from build123d import *

# Parameters (mm, degrees)
F0_W     = 30.5993435904
F0_H     = 25.6396476179
F1_DEPTH = 40
F2_R     = 6.5677441637
F3_DEPTH = 25.6406476179
F4_R     = 5
F5_SIZE  = 5
F6_T     = -2.5


with BuildPart() as f1:
    # F0 (on Top) → F1 (new body)
    with BuildSketch(Plane.XY):
        with Locations((-1.0232594796, 2.7313483879)):
            Rectangle(F0_W, F0_H)
    extrude(amount=F1_DEPTH)

    # F2 (on face) → F3 (cut, through all)
    with BuildSketch(Plane.XZ.offset(10.0884754211)):
        with Locations((-5.0276978873, 21.8645650893)):
            Circle(F2_R)
    extrude(amount=-F3_DEPTH, mode=Mode.SUBTRACT)

    # F4
    f4_edges = [f1.edges().sort_by_distance(p)[0] for p in [
        (-1.023259, -10.088475, 40),
    ]]
    fillet(f4_edges, radius=F4_R)

    # F5
    f5_edges = [f1.edges().sort_by_distance(p)[0] for p in [
        (-1.023259, 15.551172, 40),
    ]]
    chamfer(f5_edges, length=F5_SIZE)

    # F6
    f6_openings = [f1.faces().sort_by_distance(p)[0] for p in [
        (-1.023259, 2.731348, 0),
        (14.276412, 2.655308, 19.672056),
    ]]
    offset(amount=F6_T, openings=f6_openings)

    # F7: F1 across face


with BuildPart() as f1_1:
    add(f1.part)
    add(f1.part.mirror(Plane(origin=(14.2764123157, 2.5963156979, 23.1564866068), x_dir=(0, 1, 0), z_dir=(1, 0, 0))))


solid = f1_1.part
Input: part model. Units: mm. Frame: model coordinates. A direction names the side the tool comes from. Round coordinates to 2 decimals unless told otherwise and drop trailing zeros. Order: outer loops, then holes, each group sorted by start corner. A loop starts at its lowest first (then second) coordinate and runs counter-clockwise, first axis right, second up. Notation, with made-up numbers: (28, 6) - (48, 6) arc R16 ccw to (48, 31) - close; hole circle Ø2 at (87.5, -7). An arc over 180 degrees is marked (long way). Use a Markdown table: item, result.
1. Section D-D on x = 33. Return the cut outline in (y, z).
Evaluation:
| item | result |
|---|---|
| outline | (-10.09, 0) - (-7.59, 0) - (-7.59, 12.82) - (13.05, 12.82) - (13.05, 0) - (15.55, 0) - (15.55, 15.32) - (-10.09, 15.32) - close; (-10.09, 28.41) - (15.55, 28.41) - (15.55, 35) - (10.55, 40) - (-5.09, 40) arc R5 ccw to (-10.09, 35) - close; hole (-7.59, 30.91) - (13.05, 30.91) - (13.05, 33.96) - (9.52, 37.5) - (-5.09, 37.5) arc R2.5 ccw to (-7.59, 35) - close |
2. Mould query, pull axis Y, two halves, no side actions, for faces 1 (the face through (14.67, 11.308, 35.707)), 2 (the face through (13.85, -8.66, 38.5)), 3 (the face through (35.004, 2.552, 15.453)), 4 (the face through (14.7, 13.09, 37.46)). Classes: +Y half, -Y half, draft (parallel to the pull), parting line (faces both ways), or undercut.
Evaluation:
| item | result |
|---|---|
| face 1 | undercut |
| face 2 | -Y half |
| face 3 | draft |
| face 4 | +Y half |
3. Access query for faces 5 (the face through (-13.823, 3, 10)), 6 (the face through (-10.24, 2.55, 17.87)), 7 (the face through (15, 2, 37.5)). Directions: +Z, -Z, +X, -X, +Y, -Y. A direction counts if a zero-diameter tool reaches every point of the face in a straight line with its end or side. Return the directions, or none.
Evaluation:
| item | result |
|---|---|
| face 5 | -Z |
| face 6 | +Y, -Y |
| face 7 | none |
4. Material intervals for probe 1 along Z at (x, y) = (34, 0.5); probe 2 along X at (y, z) = (7, 3.5); probe 3 along Y at (x, z) = (11.5, 9), sorted ascending.
Evaluation:
| item | result |
|---|---|
| probe 1 | 12.81 to 15.31, 28.42 to 30.92, 37.5 to 40 |
| probe 2 | -16.32 to -13.82, 42.38 to 44.88 |
| probe 3 | -10.09 to -7.59, 13.05 to 15.55 |
5. First-contact query: pin 1 (6 mm diameter, centred on x = -3.5, y = -1, fed in from -Z); pin 2 (4 mm diameter, centred on x = 0.5, y = 7.5, fed in from -Z); pin 3 (11.5 mm diameter, centred on x = 22, y = 0, fed in from -Z). Flat tips, straight axial feed; report the tip coordinate or a pass-through.
Evaluation:
| item | result |
|---|---|
| pin 1 | z = 12.8 |
| pin 2 | z = 13.51 |
| pin 3 | z = 14.92 |
6. Section A-A on x = 17. Return the cut outline in (y, z), then the cut area to 3 significant figures.
Evaluation:
| item | result |
|---|---|
| outline | (-10.09, 0) - (-7.59, 0) - (-7.59, 35) arc R2.5 cw to (-5.09, 37.5) - (9.52, 37.5) - (13.05, 33.96) - (13.05, 0) - (15.55, 0) - (15.55, 35) - (10.55, 40) - (-5.09, 40) arc R5 ccw to (-10.09, 35) - close |
| area | 241 mm^2 |
7. Section B-B on z = 11.5. Return the cut outline in (x, y), then the cut area to 3 significant figures.
Evaluation:
| item | result |
|---|---|
| outline | (-16.32, -10.09) - (44.88, -10.09) - (44.88, 15.55) - (-16.32, 15.55) - close; hole (-13.82, -7.59) - (42.38, -7.59) - (42.38, 13.05) - (-13.82, 13.05) - close |
| area | 409 mm^2 |
8. Section C-C on y = 6.5. Return the cut outline in (x, z), then the cut area to 3 significant figures.
Evaluation:
| item | result |
|---|---|
| outline | (-16.32, 0) - (-13.82, 0) - (-13.82, 19.66) arc R9.07 ccw (long way) to (-13.82, 24.07) - (-13.82, 37.5) - (42.38, 37.5) - (42.38, 24.07) arc R9.07 ccw (long way) to (42.38, 19.66) - (42.38, 0) - (44.88, 0) - (44.88, 40) - (-16.32, 40) - close; hole circle Ø13.14 at (-5.03, 21.86); hole circle Ø13.14 at (33.58, 21.86) |
| area | 584 mm^2 |
